```python
from build123d import *

# Parameters (mm, degrees)
SKETCH1_W           = 3
SKETCH1_H           = 8
SKETCH1_H_2         = 3
SKETCH1_W_2         = 8
BOSS_EXTRUDE1_DEPTH = 20
SKETCH2_R           = 2
CUT_EXTRUDE1_DEPTH  = 4
SKETCH3_R           = 2
CUT_EXTRUDE2_DEPTH  = 4
SKETCH4_W           = 3
SKETCH4_H           = 11
BOSS_EXTRUDE2_DEPTH = 20
SKETCH5_R           = 2.5
CUT_EXTRUDE3_DEPTH  = 21
FILLET1_R           = 1
SKETCH6_R           = 2.5
CUT_EXTRUDE4_DEPTH  = 4


with BuildPart() as part:
    # Sketch1 → Boss-Extrude1 (new body)
    with BuildSketch(Plane(origin=(0, 0, 0), x_dir=(0, 0, -1), z_dir=(1, 0, 0))):
        with Locations((-1.5, 7)):
            Rectangle(SKETCH1_W, SKETCH1_H)
        with Locations((-1.5, 1.5)):
            Rectangle(SKETCH1_W, SKETCH1_H_2)
        with Locations((-7, 1.5)):
            Rectangle(SKETCH1_W_2, SKETCH1_H_2)
    extrude(amount=BOSS_EXTRUDE1_DEPTH)

    # Sketch2 → Cut-Extrude1 (cut, through all)
    with BuildSketch(Plane.XY.offset(3)):
        with Locations((5, 7.5)):
            Circle(SKETCH2_R)
        with Locations((15, 7.5)):
            Circle(SKETCH2_R)
    extrude(amount=-CUT_EXTRUDE1_DEPTH, mode=Mode.SUBTRACT)

    # Sketch3 → Cut-Extrude2 (cut, through all)
    with BuildSketch(Plane(origin=(0, 3, 0), x_dir=(1, 0, 0), z_dir=(0, 1, 0))):
        with Locations((6.5, -6)):
            Circle(SKETCH3_R)
        with Locations((13.5, -6)):
            Circle(SKETCH3_R)
    extrude(amount=-CUT_EXTRUDE2_DEPTH, mode=Mode.SUBTRACT)

    # Sketch4 → Boss-Extrude2 (add)
    with BuildSketch(Plane.XZ):
        with Locations((1.5, 5.5)):
            Rectangle(SKETCH4_W, SKETCH4_H)
    extrude(amount=BOSS_EXTRUDE2_DEPTH)

    # Sketch5 → Cut-Extrude3 (cut, through all)
    with BuildSketch(Plane.ZY):
        with Locations((6, -15)):
            Circle(SKETCH5_R)
    extrude(amount=-CUT_EXTRUDE3_DEPTH, mode=Mode.SUBTRACT)

    # Fillet1
    fillet1_edges = [part.edges().sort_by_distance(p)[0] for p in [
        (20, 3, 7),
        (0, 3, 7),
        (0, 7, 3),
        (10, 11, 3),
        (10, 11, 0),
        (11.5, 0, 0),
        (11.5, 0, 11),
        (10, 3, 11),
        (20, 1.5, 11),
        (20, 0, 5.5),
        (20, 5.5, 0),
        (20, 11, 1.5),
        (3, -10, 0),
        (3, -10, 11),
        (0, -20, 5.5),
        (1.5, -20, 0),
        (3, -20, 5.5),
        (1.5, -20, 11),
        (20, 7, 3),
        (0, 11, 1.5),
        (0, -4.5, 0),
        (0, -8.5, 11),
    ]]
    fillet(fillet1_edges, radius=FILLET1_R)

    # Sketch6 → Cut-Extrude4 (cut, through all)
    with BuildSketch(Plane(origin=(3, 0, 0), x_dir=(0, 0, -1), z_dir=(1, 0, 0))):
        with Locations((-5.5, -7)):
            Circle(SKETCH6_R)
    extrude(amount=-CUT_EXTRUDE4_DEPTH, mode=Mode.SUBTRACT)


solid = part.part
```
Geometry check sheet. Reference: the model listing, model coordinates, mm. A direction names the side the tool comes from. Round coordinates to 2 decimals unless told otherwise and drop trailing zeros. Loops run counter-clockwise (first coordinate to the right, second up) from the corner with the lowest first, then second, coordinate; pieces in that order, holes last. Notation, with made-up numbers: (77, 32.5) - (128, 32.5) arc R32 ccw to (128, 63.5) - close; hole circle Ø5 at (-29, 53). An arc over 180 degrees is marked (long way). Use a Markdown table: item, result.
Q1. Draft check along Z on faces 6 (the cylindrical face through (1.52, -7.96, 3.19)), 7 (the cylindrical face through (0.285, -8.353, 10.699)), 8 (the cylindrical face through (0.285, -4.703, 0.301)), 9 (the flat face through (3, -9, 3)). Enter one of: released by +Z, released by -Z, zero draft, split by the parting line, or undercut.
Solutions:
| item | result |
|---|---|
| face 6 | undercut |
| face 7 | released by +Z |
| face 8 | released by -Z |
| face 9 | zero draft |
Q2. Cross-section at D-D on z = 5.5. Record the cut outline in (x, y).
Solutions:
| item | result |
|---|---|
| outline | (0, -19) arc R1 ccw to (1, -20) - (2, -20) arc R1 ccw to (3, -19) - (3, -17.45) - (0, -17.45) - close; (0, -12.55) - (3, -12.55) - (3, -9.5) - (0, -9.5) - close; (0, -4.5) - (3, -4.5) - (3, 0) - (4.56, 0) - (4.56, 3) - (1, 3) arc R1 ccw to (0, 2) - close; (8.44, 0) - (11.56, 0) - (11.56, 3) - (8.44, 3) - close; (15.44, 0) - (19, 0) arc R1 ccw to (20, 1) - (20, 2) arc R1 ccw to (19, 3) - (15.44, 3) - close |
Q3. Cross-section at B-B on y = 7.5. Record the cut outline in (x, z), plus the area to 3 significant figures.
Solutions:
| item | result |
|---|---|
| outline | (0, 1) arc R1 ccw to (1, 0) - (3, 0) - (3, 3) - (1, 3) arc R1 ccw to (0, 2) - close; (7, 0) - (13, 0) - (13, 3) - (7, 3) - close; (17, 0) - (19, 0) arc R1 ccw to (20, 1) - (20, 2) arc R1 ccw to (19, 3) - (17, 3) - close |
| area | 35.1 mm2 |
Q4. Access from +Z, -Z, +X, -X, +Y, -Y to the whole of each face (thin tool, end or side, straight path). Record for faces 1 (the flat face through (10, 7, 3)), 2 (the cylindrical face through (0.285, 2.699, 5.944)), 3 (the flat face through (1.3, -5.3, 11)), 4 (the cylindrical face through (10.619, 0.301, 0.285)), 5 (the cylindrical face through (10.619, 0.301, 10.715)).
Solutions:
| item | result |
|---|---|
| face 1 | +Z, +X, -X, +Y |
| face 2 | +Z, -X, +Y |
| face 3 | +Z, +X, -X, +Y, -Y |
| face 4 | -Z, +X, -Y |
| face 5 | +Z, +X, -Y |
Q5. Material ranges on line 1 (X direction, y = 1.8, z = 6); line 2 (Y direction, x = 15, z = 1.05); line 3 (Y direction, x = 1.35, z = 5.5), recorded low to high.
Solutions:
| item | result |
|---|---|
| line 1 | x = 0 to 4.5, 8.5 to 11.5, 15.5 to 20 |
| line 2 | y = 0 to 5.5, 9.5 to 11 |
| line 3 | y = -20 to -17.45, -12.55 to -9.5, -4.5 to 3 |
Q6. Go/stop test with flat-tipped pins: P1, Ø3, axis at y = -8, z = 2.5, coming from the +X side; P2, Ø4, axis at x = 5.5, y = 8, coming from the -Z side; P3, Ø7.5, axis at x = 12, y = 6, coming from the +Z side; P4, Ø4.5, axis at x = 15, y = 7.5, coming from the +Z side. Record where each tip stops, or that it passes through.
Solutions:
| item | result |
|---|---|
| P1 | stops at x = 3 |
| P2 | stops at z = 0 |
| P3 | stops at z = 10.97 |
| P4 | stops at z = 3 |
Q7. Cross-section at A-A on y = -7. Record the cut outline in (x, z).
Solutions:
| item | result |
|---|---|
| outline | (0, 1) arc R1 ccw to (1, 0) - (2, 0) arc R1 ccw to (3, 1) - (3, 3) - (0, 3) - close; (0, 8) - (3, 8) - (3, 10) arc R1 ccw to (2, 11) - (1, 11) arc R1 ccw to (0, 10) - close |
Q8. Cross-section at C-C on z = 9.5. Record the cut outline in (x, y).
Solutions:
| item | result |
|---|---|
| outline | (0, -19) arc R1 ccw to (1, -20) - (2, -20) arc R1 ccw to (3, -19) - (3, 0) - (19, 0) arc R1 ccw to (20, 1) - (20, 2) arc R1 ccw to (19, 3) - (1, 3) arc R1 ccw to (0, 2) - close |
